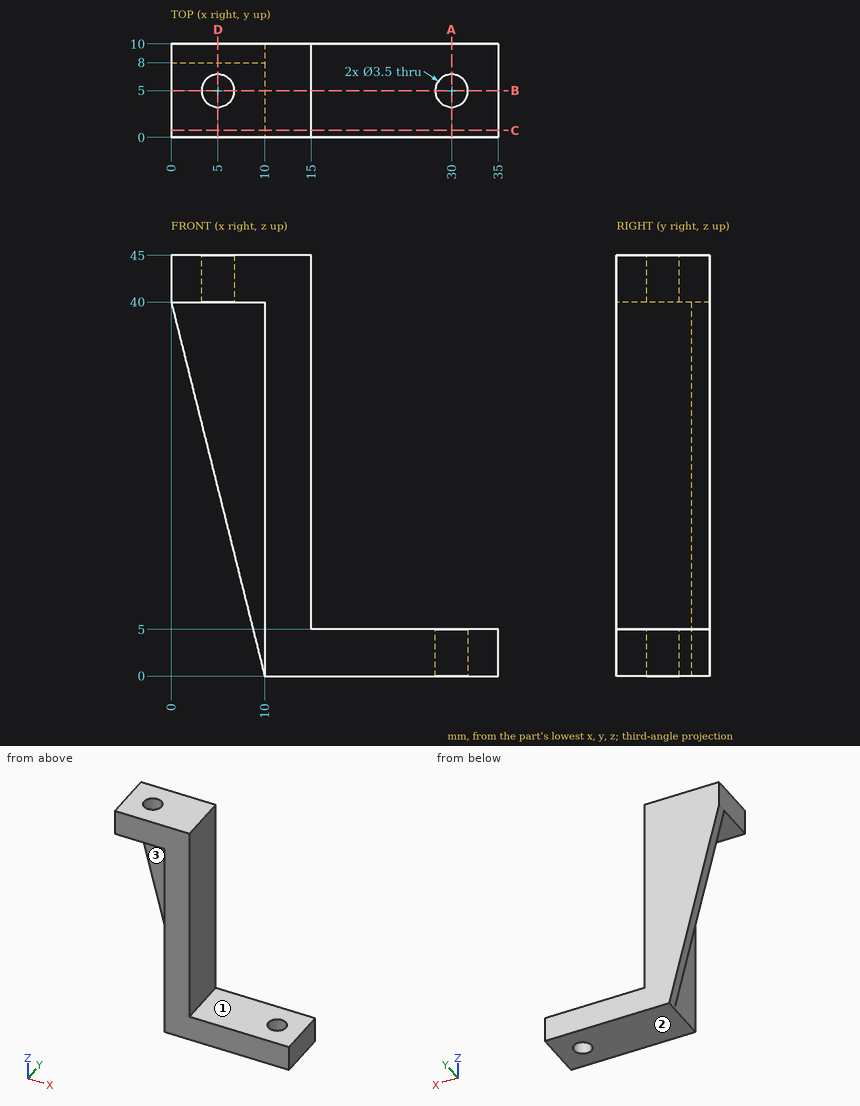
Print and shaded views of the part. All mm, measured from the part's lowest x, y and z. A direction names the side the tool comes from. Coordinates: 2 decimals unless noted, no trailing zeros. Order: outer loops, then holes, each group sorted by start corner. A loop starts at its lowest first (then second) coordinate and runs counter-clockwise, first axis right, second up. Notation, with made-up numbers: (38.25, 14) -> (94.25, 14) arc R16 cw to (94.25, 37) -> close; hole circle Ø8 at (-20, -8.5). An arc over 180 degrees is marked (long way). Answer as a JSON object with one key per item and string values. Group by question number.
1) Drill centre lines: L1, parallel to Y at x = 5, z = 41; L2, parallel to X at y = 6, z = 13.5; L3, parallel to Z at x = 26.5, y = 0.5. Where is each one in solid material? Low to high.
2) Flat gauge pins, fed straight in: pin 1 (6 mm diameter, centred on x = 21, y = 8.5, fed in from -Z); pin 2 (6 mm diameter, centred on y = 7, z = 9, fed in from +X); pin 3 (4 mm diameter, centred on x = 5, y = 4, fed in from -Z); pin 4 (2.5 mm diameter, centred on y = 5.5, z = 30, fed in from -X). Where does each tip first touch, or does it go through?
3) Cut at D-D, the plane x = 5. Write the cut outline in (y, z), then the cut area to 3 significant figures.
4) Cut at C-C, the plane y = 0.75. Write the cut outline in (x, z).
5) Cut at A-A, the plane x = 30. Write the cut outline in (y, z).
6) Which spindle directions (+Z, -Z, +X, -X, +Y, -Y) get a long thin tool onto all of the face, cutting with end or side? Do the marked faces 1, 2 and 3. Say none if no direction does.
7) Cut at B-B, the plane y = 5. Write the cut outline in (x, z), then the cut area to 3 significant figures.
Check values:
{
 "1": {"L1": "y = 0 to 3.25, 6.75 to 10", "L2": "x = 10 to 15", "L3": "z = 0 to 5"},
 "2": {"pin 1": "stops at z = 0", "pin 2": "stops at x = 15", "pin 3": "stops at z = 40", "pin 4": "stops at x = 10"},
 "3": {"outline": "(0, 40) -> (3.25, 40) -> (3.25, 45) -> (0, 45) -> close; (6.75, 40) -> (8, 40) -> (8, 20) -> (10, 20) -> (10, 45) -> (6.75, 45) -> close", "area": "72.5 mm²"},
 "4": {"outline": "(0, 40) -> (10, 40) -> (10, 0) -> (35, 0) -> (35, 5) -> (15, 5) -> (15, 45) -> (0, 45) -> close"},
 "5": {"outline": "(0, 0) -> (3.25, 0) -> (3.25, 5) -> (0, 5) -> close; (6.75, 0) -> (10, 0) -> (10, 5) -> (6.75, 5) -> close"},
 "6": {"face 1": "+Z, +X, +Y, -Y", "face 2": "-Z, +X, -X, +Y, -Y", "face 3": "-Z, -X, -Y"},
 "7": {"outline": "(0, 40) -> (3.25, 40) -> (3.25, 45) -> (0, 45) -> close; (6.75, 40) -> (10, 40) -> (10, 0) -> (28.25, 0) -> (28.25, 5) -> (15, 5) -> (15, 45) -> (6.75, 45) -> close; (31.75, 0) -> (35, 0) -> (35, 5) -> (31.75, 5) -> close", "area": "340 mm²"}
}
